Print and shaded views of the part. All mm, measured from the part's lowest x, y and z. Give positions to 0.01 mm unless a question says otherwise; leave off trailing zeros. Answer in a Markdown table with one row per item.
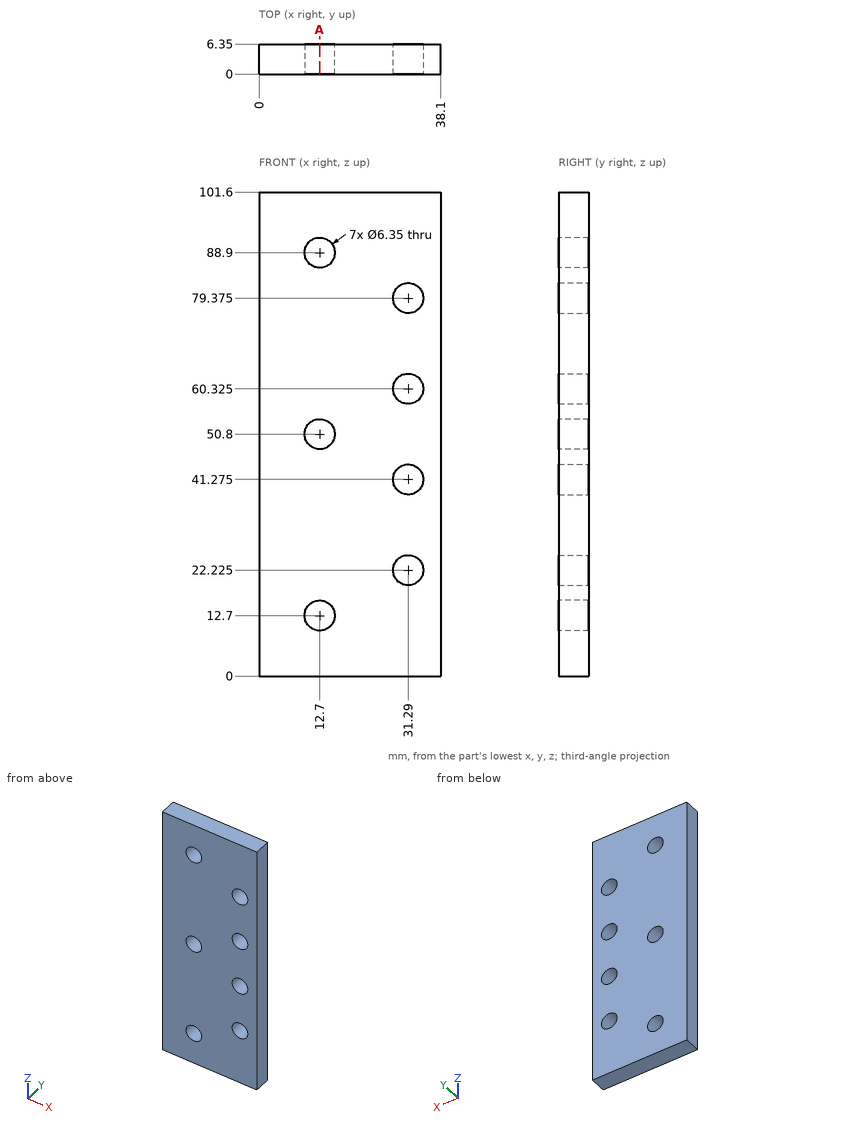
1. Probe line 1 (Z direction, x = 12.7, y = 3.25) (1 decimal); line 2 (X direction, y = 5, z = 88.9) (1 decimal); line 3 (Z direction, x = 13.5, y = 5). List the from-to ranges inside material, lowest first.
Check result:
| item | result |
|---|---|
| line 1 | z = 0 to 9.5, 15.9 to 47.6, 54 to 85.7, 92.1 to 101.6 |
| line 2 | x = 0 to 9.5, 15.9 to 38.1 |
| line 3 | z = 0 to 9.63, 15.77 to 47.73, 53.87 to 85.83, 91.97 to 101.6 |
2. Cut at A-A on x = 12.7. Count the separate pieces of the cut face and the enclosed holes in it, and give its area (3 significant figures).
Check result:
| item | result |
|---|---|
| separate pieces | 4 |
| enclosed holes | 0 |
| area | 524 mm² |
3. Drop a flat-ended pin along its axis: P1, Ø5, axis at x = 31.29, z = 22.22, coming from the -Y side. Give the stop position or say it passes through.
Check result:
| item | result |
|---|---|
| P1 | passes through |
